Can you work these out from the model? Positions are in its coordinate system, mm. A direction names the side the tool comes from. Coordinates: 2 decimals unless noted, no trailing zeros. Loops run counter-clockwise (first coordinate to the right, second up) from the corner with the lowest first, then second, coordinate; pieces in that order, holes last. Notation, with made-up numbers: (67.5, -26) - (79.5, -26) arc R20 ccw to (79.5, -3) - close; hole circle Ø9 at (28.25, -38). An arc over 180 degrees is marked (long way). Put each result on its own line as item: value. Start each with the question number.
Autodesk Inventor part; units mm, degrees
ref_plane "YZ Plane" through (0, 0, 0) normal (1, 0, 0) x (0, 1, 0)
ref_plane "XZ Plane" through (0, 0, 0) normal (0, 1, 0) x (-1, 0, 0)
ref_plane "XY Plane" through (0, 0, 0) normal (0, 0, 1) x (1, 0, 0)
sketch "Sketch1" plane through (0, 0, 0) normal (0, 0, 1) x (1, 0, 0)
  line L0 (3.0839, 107.4917) -> (15.7839, 107.4917)
  line L1 (15.7839, 107.4917) -> (15.7839, -0.4583)
  line L2 (15.7839, -0.4583) -> (3.0839, -0.4583)
  line L3 (3.0839, -0.4583) -> (3.0839, 107.4917)
  line L4 (33.221, 2.0817) -> (3.0839, 2.0817)
  line L5 (33.221, 14.8071) -> (3.0839, 14.8071)
  line L6 (15.7839, -0.4583) -> (33.221, -0.4583)
  line L7 (33.221, -0.4583) -> (33.221, 17.3471)
  line L8 (33.221, 17.3471) -> (15.7839, 17.3471)
  circle A0 centre (28.776, 8.4444) radius 2.159
  circle A1 centre (9.726, 8.4444) radius 2.159
  line L9 (9.726, 6.2854) -> (28.776, 6.2854)
  line L10 (9.726, 10.6034) -> (28.776, 10.6034)
  point P0 (9.4212, 101.1417)
  point P1 (9.4212, 88.4417)
  point P2 (9.4212, 75.7417)
  point P3 (15.7839, 2.0817)
  point P4 (15.7839, 14.8071)
  dimension "d0" = 12.7
  dimension "d1" = 107.95
  dimension "d2" = 6.35
  dimension "d3" = 12.7
  dimension "d4" = 6.3626
  dimension "d5" = 6.3626
  dimension "d6" = 6.3626
  dimension "d7" = 12.7
  dimension "d17" = 2.54
  dimension "d18" = 12.7254
  dimension "d21" = 17.4371
  dimension "d22" = 2.54
  dimension "d23" = 4.318
  dimension "d24" = 6.3627
  dimension "d25" = 4.445
  dimension "d26" = 4.318
  dimension "d27" = 6.3627
  dimension "d28" = 19.05
extrude "Extrusion1" add sketch "Sketch1" along normal blind 12.7
hole "Hole1" at (9.4212, 101.1417, 0) at (9.4212, 88.4417, 0) at (9.4212, 75.7417, 0) direction (0, 0, 1) diameter 6.5278 end through all counterbore diameter 11.1252 counterbore depth 6.35
extrude "Extrusion2" cut sketch "Sketch1" along normal blind 3.81 contours L5 L1 L10 A1 L9 L4 L3 | L5 L7 L4 L1 L9 A0 L10 | L10 A0 L9 L1 | L1 L9 A1 L10 | A1 | A0
extrude "Extrusion3" cut sketch "Sketch1" along normal through all contours L10 A0 L9 L1 | L1 L9 A1 L10 | A1 | A0
equation "\"d29\" = d27"
properties part number "J005772" material "STAINLESS STEEL, 17-4, H900"
Q1. I want a section at D-D on y = 53.5. List the corners of the cut face in (x, z) for me, and give its area (3 significant figures).
Q2. I want a section at A-A on x = 17. List the corners of the cut face in (y, z) for me, and give its area (3 significant figures).
Q3. On a 3-axis mill with a long thin cutter (end or side, diameter ignored), from which of +Z, -Z, +X, -X, +Y, -Y can I reach the whole of each face in a straight line? I mean faces 1 (the flat face through (25, 17.347, 6)), 2 (the cylindrical face through (11.55, 93.58, 3.22)), 3 (the flat face through (19, 10.603, 8)). Say none if no direction works.
Q4. I want a section at B-B on z = 2.5. List the corners of the cut face in (x, y) for me.
Q5. I want a section at C-C on z = 8.5. List the corners of the cut face in (x, y) for me.
Q6. Will these pins go through, and if not, where does the flat tip stop? pin 1 (4 mm diameter, centred on y = 86, z = 11, fed in from +X); pin 2 (6 mm diameter, centred on x = 9.42, y = 101.14, fed in from +Z); pin 3 (6.5 mm diameter, centred on x = 21, z = 4.5, fed in from +Y).
Q7. Please list where these lines run through material, in increasing order: line 1 along Y through (x, z) = (9.5, 9.5); line 2 along Y through (x, z) = (14.5, 8); line 3 along Y through (x, z) = (24, 8.75). Write a range as [from, to].
Q8. We'd pull the mould along X, two halves only. Please class faces 4 (the cylindrical face through (7.568, 8.397, 8.193)), 5 (the flat face through (15.784, 63, 6)), 6 (the flat face through (13, 51, 0)): released by +X, released by -X, zero draft, split by the parting line, or undercut.
Calculated:
1. outline: (3.08, 0) - (15.78, 0) - (15.78, 12.7) - (3.08, 12.7) - close
1. area: 161 mm2
2. outline: (-0.46, 0) - (2.08, 0) - (2.08, 3.81) - (6.29, 3.81) - (6.29, 12.7) - (-0.46, 12.7) - close; (10.6, 3.81) - (14.81, 3.81) - (14.81, 0) - (17.35, 0) - (17.35, 12.7) - (10.6, 12.7) - close
2. area: 139 mm2
3. face 1: +Z, -Z, +X, +Y
3. face 2: -Z
3. face 3: +Z, -Z
4. outline: (3.08, -0.46) - (33.22, -0.46) - (33.22, 2.08) - (3.08, 2.08) - close; (3.08, 14.81) - (33.22, 14.81) - (33.22, 17.35) - (15.78, 17.35) - (15.78, 107.49) - (3.08, 107.49) - close; hole circle Ø11.13 at (9.42, 75.74); hole circle Ø11.13 at (9.42, 88.44); hole circle Ø11.13 at (9.42, 101.14)
5. outline: (3.08, -0.46) - (33.22, -0.46) - (33.22, 17.35) - (15.78, 17.35) - (15.78, 107.49) - (3.08, 107.49) - close; hole circle Ø6.53 at (9.42, 75.74); hole circle Ø6.53 at (9.42, 88.44); hole circle Ø6.53 at (9.42, 101.14); hole (9.73, 6.29) - (28.78, 6.29) arc R2.16 ccw to (28.78, 10.6) - (9.73, 10.6) arc R2.16 ccw to start
6. pin 1: x = 15.78
6. pin 2: through
6. pin 3: y = 17.35
7. line 1: [-0.46, 6.3], [10.59, 72.48], [79, 85.18], [91.7, 97.88], [104.4, 107.49]
7. line 2: [-0.46, 6.29], [10.6, 107.49]
7. line 3: [-0.46, 6.29], [10.6, 17.35]
8. face 4: undercut
8. face 5: released by +X
8. face 6: zero draft
